Part model, mm, in its own coordinate system. A direction names the side the tool comes from. Coordinates: 2 decimals unless noted, no trailing zeros. Write each loop counter-clockwise with the first axis right and the second up, starting at its lowest first coordinate (ties: lowest second). Pieces come first, ordered by that corner, then holes. Notation, with made-up numbers: (-19, 7) -> (25, 7) arc R28 cw to (25, 30) -> close; hole circle Ø11 at (41, 86.5). An arc over 180 degrees is marked (long way). One line per question, with ' | ' between items. Start each with the question number.
Item 1: Two-plate mould, pull along Z, no slides. Class faces 1 (the cylindrical face through (-0.03, 21.9, 18.03)), 2 (the flat face through (1, 18.6, 16)), 3 (the cylindrical face through (-0.028, 26.283, 10.74)), 4 (the cylindrical face through (0, -10.7, 10.9)): pulls with the +Z half, pulls with the -Z half, needs draft (parallel to the pull), parting line crosses it, or undercut.
Item 2: Saw through at D-D (y = -5.7). List the corners of the cut face in (x, z), and give its area (3 significant figures).
Item 3: 3-axis set-ups, long thin cutter, end or side, ignore diameter. For faces 5 (the flat face through (2, 0.5, 15.8)), 6 (the flat face through (2, -3.5, 11.2)), 7 (the flat face through (3, 1, 16)): which of +Z, -Z, +X, -X, +Y, -Y reach the whole face in a straight line?
Item 4: Saw through at A-A (z = 11). List the corners of the cut face in (x, y).
Item 5: Probe probe 1 along Y at (x, z) = (0.6, 11); probe 2 along Y at (x, z) = (-1.2, 11); probe 3 along Y at (x, z) = (3, 20.5). List the from-to ranges inside material, lowest first. Write a range as [from, to].
Item 6: Saw through at B-B (z = 23). List the corners of the cut face in (x, y).
Item 7: Saw through at C-C (x = -1.2). List the corners of the cut face in (y, z), and give its area (3 significant figures).
Item 8: Pin check, flat tips, straight feed: pin 1 (9.5 mm diameter, centred on y = -8.5, z = 11.5, fed in from +X); pin 2 (0.6 mm diameter, centred on x = 3, z = 17, fed in from -Y); pin 3 (0.6 mm diameter, centred on x = 1, z = 18, fed in from -Y). Stop position of each tip, or through.
from build123d import *

# Parameters (mm, degrees)
BOSS_EXTRU_1_DEPTH = 32
ESQUISSE2_R        = 2
BOSS_EXTRU_2_DEPTH = 4
CONG_1_R           = 6


with BuildPart() as part:
    # Esquisse1 → Boss.-Extru.1 (new body)
    with BuildSketch(Plane.XY):
        Polygon((4, -2), (4, 1), (2, 1), (2, 0), (0, 0), (0, 18.6), (2, 18.6), (2, 17.6), (4, 17.6), (4, 20.6), (-2, 20.6), (-2, -2), align=None)
    extrude(amount=BOSS_EXTRU_1_DEPTH)

    # Esquisse2 → Boss.-Extru.2 (add)
    # profile 1 of 2: a face of its own
    with BuildSketch(Plane.ZY.offset(2)):
        with BuildLine():
            Line((6, -2), (6, -5.7))
            ThreePointArc((6, -5.7), (11, -10.7), (16, -5.7))
            Line((16, -5.7), (16, -2))
            Line((16, -2), (6, -2))
        make_face()
        with Locations((11, -5.7)):
            Circle(ESQUISSE2_R, mode=Mode.SUBTRACT)
    # profile 2 of 2: a face of its own
    with BuildSketch(Plane.ZY.offset(2)):
        with BuildLine():
            Line((6, 20.6), (6, 24.3))
            ThreePointArc((6, 24.3), (11, 29.3), (16, 24.3))
            Line((16, 24.3), (16, 20.6))
            Line((16, 20.6), (6, 20.6))
        make_face()
        with Locations((11, 24.3)):
            Circle(ESQUISSE2_R, mode=Mode.SUBTRACT)
    extrude(amount=-BOSS_EXTRU_2_DEPTH)

    # Congé1
    # the kernel refuses this fillet: 6 mm, written as the material it adds along each edge
    with BuildSketch(Plane(origin=(-2, -2, 16), x_dir=(0, 0, 1), z_dir=(1, 0, 0)), Plane(origin=(-2, 20.6, 6), x_dir=(0, 0, -1), z_dir=(1, 0, 0))) as cong_1_piece_1:
        with BuildLine():
            CenterArc((5.756858277, 6), CONG_1_R, 192.069082524, 77.930917476)
            Line((-0.110518965, 4.745454545), (-0.697256689, 4.62))
            ThreePointArc((-0.697256689, 4.62), (-0.6, 3.7), (-0.6, 0))
            Line((-0.6, 0), (0, -0.6))
            Line((0, -0.6), (5.756858277, -0.6))
            Line((5.756858277, -0.6), (5.756858277, 0))
        make_face()
    extrude(amount=4)
    with BuildSketch(Plane(origin=(-2, 20.6, 16), x_dir=(0, 0, 1), z_dir=(1, 0, 0)), Plane(origin=(-2, -2, 6), x_dir=(0, 0, -1), z_dir=(1, 0, 0))) as cong_1_piece_2:
        with BuildLine():
            CenterArc((5.756858277, -6), CONG_1_R, 90, 77.930917476)
            Line((-0.110518965, -4.745454545), (-0.697256689, -4.62))
            ThreePointArc((-0.697256689, -4.62), (-0.6, -3.7), (-0.6, 0))
            Line((-0.6, 0), (0, 0.6))
            Line((0, 0.6), (5.756858277, 0.6))
            Line((5.756858277, 0.6), (5.756858277, 0))
        make_face()
    extrude(amount=4)


solid = part.part
From the geometry:
1) face 1: pulls with the +Z half | face 2: needs draft | face 3: undercut | face 4: parting line crosses it
2) outline: (-2, 5.78) -> (2, 5.78) -> (2, 9) -> (-2, 9) -> close; (-2, 13) -> (2, 13) -> (2, 16.22) -> (-2, 16.22) -> close | area: 25.7 mm2
3) face 5: +Z, -Z | face 6: +Z, -Z, +X, -Y | face 7: +Z, -Z, +X
4) outline: (-2, -10.7) -> (2, -10.7) -> (2, -7.7) -> (-2, -7.7) -> close; (-2, -3.7) -> (2, -3.7) -> (2, -2) -> (4, -2) -> (4, 1) -> (2, 1) -> (2, 0) -> (0, 0) -> (0, 18.6) -> (2, 18.6) -> (2, 17.6) -> (4, 17.6) -> (4, 20.6) -> (2, 20.6) -> (2, 22.3) -> (-2, 22.3) -> close; (-2, 26.3) -> (2, 26.3) -> (2, 29.3) -> (-2, 29.3) -> close
5) probe 1: [-10.7, -7.7], [-3.7, 0], [18.6, 22.3], [26.3, 29.3] | probe 2: [-10.7, -7.7], [-3.7, 22.3], [26.3, 29.3] | probe 3: [-2, 1], [17.6, 20.6]
6) outline: (-2, -2) -> (4, -2) -> (4, 1) -> (2, 1) -> (2, 0) -> (0, 0) -> (0, 18.6) -> (2, 18.6) -> (2, 17.6) -> (4, 17.6) -> (4, 20.6) -> (-2, 20.6) -> close
7) outline: (-6.75, 6.11) arc R6 cw to (-2, 0.24) -> (-2, 0) -> (20.6, 0) -> (20.6, 0.24) arc R6 cw to (25.35, 6.11) arc R5 ccw to (25.35, 15.89) arc R6 cw to (20.6, 21.76) -> (20.6, 32) -> (-2, 32) -> (-2, 21.76) arc R6 cw to (-6.75, 15.89) arc R5 ccw to start; hole circle Ø4 at (-5.7, 11); hole circle Ø4 at (24.3, 11) | area: 877 mm2
8) pin 1: x = 2 | pin 2: y = -2 | pin 3: y = -3.58
